```python
from build123d import *

# Parameters (mm, degrees)
F0_W     = 114.3
F0_H     = 10.16
F1_DEPTH = 12.2174
F2_W     = 114.3
F2_H     = 2.794
F3_DEPTH = 8.3566
F4_R     = 1.905
F5_DEPTH = 25.4


with BuildPart() as f1:
    # F0 (on Front) → F1 (new body)
    with BuildSketch(Plane.XZ):
        Rectangle(F0_W, F0_H)
    extrude(amount=F1_DEPTH)

    # F2 (on face) → F3 (cut)
    with BuildSketch(Plane.XY.offset(5.08)):
        with Locations((0, -6.303842)):
            Rectangle(F2_W, F2_H)
    extrude(amount=-F3_DEPTH, mode=Mode.SUBTRACT)

    # F4 (on face) → F5 (cut)
    with BuildSketch(Plane.XZ.offset(12.2174)):
        with Locations((-50.835151, 0)):
            Circle(F4_R)
        with Locations((51.921636, 0)):
            Circle(F4_R)
    extrude(amount=-F5_DEPTH, mode=Mode.SUBTRACT)


solid = f1.part
```
Part model, mm, in its own coordinate system. A direction names the side the tool comes from. Round coordinates to 2 decimals unless told otherwise and drop trailing zeros. Write each loop counter-clockwise with the first axis right and the second up, starting at its lowest first coordinate (ties: lowest second). Pieces come first, ordered by that corner, then holes. Notation, with made-up numbers: M -27,-33 L 17,-33 A19 ccw 17,-15 Z; hole C 3.25,73 d1. An arc over 180 degrees is marked long. One line per question, with ' | ' between items.
(1) Two-plate mould, pull along Y, no slides. Class faces 1 (the face through (-1, -2, 5.08)), 2 (the face through (-1, -4.907, 1)), 3 (the face through (-1, -12.217, 0)): released by +Y, released by -Y, zero draft, split by the parting line, or undercut.
Answer key:
face 1: zero draft | face 2: undercut | face 3: released by -Y
(2) Saw through at C-C on x = 23.5. Write the cut outline in (y, z), then the cut area to 3 significant figures.
Answer key:
outline: M -12.22,-5.08 L 0,-5.08 L 0,5.08 L -4.91,5.08 L -4.91,-3.28 L -7.7,-3.28 L -7.7,5.08 L -12.22,5.08 Z | area: 101 mm^2
(3) Saw through at A-A on z = 0. Write the cut outline in (x, y).
Answer key:
outline: M -57.15,-12.22 L -52.74,-12.22 L -52.74,-7.7 L -57.15,-7.7 Z; M -57.15,-4.91 L -52.74,-4.91 L -52.74,0 L -57.15,0 Z; M -48.93,-12.22 L 50.02,-12.22 L 50.02,-7.7 L -48.93,-7.7 Z; M -48.93,-4.91 L 50.02,-4.91 L 50.02,0 L -48.93,0 Z; M 53.83,-12.22 L 57.15,-12.22 L 57.15,-7.7 L 53.83,-7.7 Z; M 53.83,-4.91 L 57.15,-4.91 L 57.15,0 L 53.83,0 Z
(4) 3-axis set-ups, long thin cutter, end or side, ignore diameter. For faces 4 (the face through (-1, -6, -3.277)), 5 (the face through (-1, 0, 0)): which of +Z, -Z, +X, -X, +Y, -Y reach the whole face in a straight line?
Answer key:
face 4: +Z, +X, -X | face 5: +Z, -Z, +X, -X, +Y
(5) Pin check, flat tips, straight feed: pin 1 (1.5 mm diameter, centred on x = 44.5, z = 2, fed in from +Y); pin 2 (1.4 mm diameter, centred on x = 14.5, y = -6, fed in from +Z). Stop position of each tip, or through.
Answer key:
pin 1: stops at y = 0 | pin 2: stops at z = -3.28
(6) Saw through at B-B on y = -11.25. Write the cut outline in (x, z) (3 decimals).
Answer key:
outline: M -57.15,-5.08 L 57.15,-5.08 L 57.15,5.08 L -57.15,5.08 Z; hole C -50.835,0 d3.81; hole C 51.922,0 d3.81
(7) Probe line 1 along Y through (x, z) = (25.5, 4); line 2 along X through (y, z) = (-1.5, -1.5); line 3 along X through (y, z) = (-8.5, -1.75). List the from-to ranges inside material, lowest first.
Answer key:
line 1: y = -12.22 to -7.7, -4.91 to 0 | line 2: x = -57.15 to -52.01, -49.66 to 50.75, 53.1 to 57.15 | line 3: x = -57.15 to -51.59, -50.08 to 51.17, 52.67 to 57.15
